The model under review builds one solid part; all positions refer to its coordinate system, in mm. Give positions to 0.01 mm unless a question says otherwise; leave off trailing zeros. Order: outer loops, then holes, each group sorted by start corner. A loop starts at its lowest first (then second) coordinate and runs counter-clockwise, first axis right, second up. Notation, with made-up numbers: (86, 39.25) - (134, 39.25) arc R27 cw to (134, 55.25) - close; hole circle Ø3 at (81, -38.75). An arc over 180 degrees is marked (long way). Use a Markdown table: item, result. Add a question column.
Autodesk Fusion 360 part; units mm, degrees
sketch "草图1" plane through (0, 0, 0) normal (0, 1, 0) x (1, 0, 0)
  line L0 (-18.7279, -36.0337) -> (2.3028, -15.3397)
  line L1 (2.3028, -15.3397) -> (28.4829, -28.9463)
  line L2 (28.4829, -28.9463) -> (15.3006, -2.5501)
  line L3 (15.3006, -2.5501) -> (36.3313, 18.1439)
  line L4 (7.1534, 13.7637) -> (36.3313, 18.1439)
  line L5 (7.1534, 13.7637) -> (-6.0289, 40.1599)
  line L6 (-6.0289, 40.1599) -> (-10.8795, 11.0565)
  line L7 (-40.0574, 6.6762) -> (-10.8795, 11.0565)
  line L8 (-40.0574, 6.6762) -> (-13.8773, -6.9304)
  line L9 (-13.8773, -6.9304) -> (-18.7279, -36.0337)
  line L10 (-30.4812, 5.0802) -> (-12.8573, 7.726)
  line L11 (10.0219, 11.1607) -> (27.6459, 13.8065)
  line L12 (-4.5877, 30.5593) -> (-7.5175, 12.9803)
  line L13 (-11.321, -9.8405) -> (-14.2508, -27.4195)
  line L14 (-30.4812, 5.0802) -> (-14.668, -3.1384)
  line L15 (5.8605, -13.8078) -> (21.6738, -22.0264)
  line L16 (-14.2508, -27.4195) -> (-1.5478, -14.9199)
  line L17 (14.943, 1.3069) -> (27.6459, 13.8065)
  line L18 (21.6738, -22.0264) -> (13.7114, -6.0826)
  line L19 (3.3747, 14.6154) -> (-4.5877, 30.5593)
  circle A0 centre (0, 0) radius 11
  arc A1 (-12.8573, 7.726) -> (-14.668, -3.1384) centre (0, 0) ccw
  arc A2 (3.3747, 14.6154) -> (-7.5175, 12.9803) centre (0, 0) ccw
  arc A3 (14.943, 1.3069) -> (10.0219, 11.1607) centre (0, 0) ccw
  arc A4 (-11.321, -9.8405) -> (-1.5478, -14.9199) centre (0, 0) ccw
  arc A5 (5.8605, -13.8078) -> (13.7114, -6.0826) centre (0, 0) ccw
  dimension "d3" = 30
  dimension "d8" = 22
sketch "草图3" plane through (0, 0, 0) normal (0, 1, 0) x (1, 0, 0)
  circle A0 centre (-75, 0) radius 2.5
  circle A1 centre (-75, 0) radius 4
  dimension "d4" = 5
  dimension "d5" = 8
extrude "拉伸1" add sketch "草图3" along normal blind 3 makes body 1
extrude "拉伸2" add sketch "草图1" along normal blind 3 separate body makes body 2
move_body "移动1" bodies 1 to x (1, 0, 0) y (0, 1, 0) z (0, 0, 1) at (69.0763, 0, -40.5763)
move_body "移动2" bodies 1 to x (1, 0, 0) y (0, 1, 0) z (0, 0, 1) at (-0.4652, 0, -2.1709)
combine "合并1" operation add target body 2 tool bodies 1
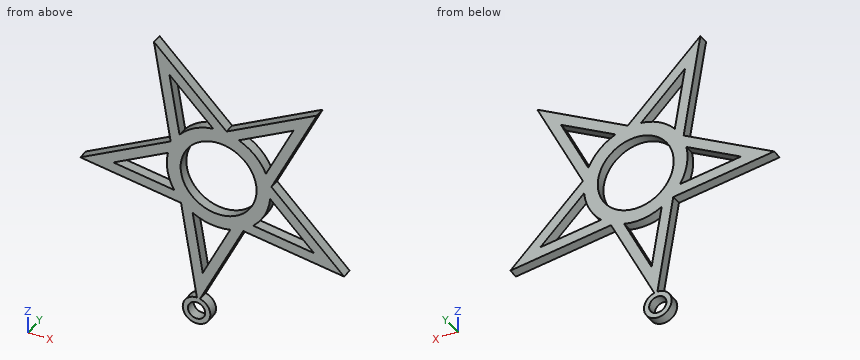
Q1. We need section C-C (z = 0). Write out the cut boundary in (x, y), plus the area to 3 significant figures.
Q2. We need section D-D (z = 16.5). Write out the cut boundary in (x, y).
Q3. We need section B-B (x = 0). Write out the cut boundary in (y, z).
Q4. Clearance check with flat-ended pins moving along their axes: P1, Ø17.5, axis at x = 0, z = 0, coming from the +Y side; P2, Ø1, axis at x = 5, y = 0.5, coming from the +Z side; P3, Ø1, axis at x = 15, y = 0.5, coming from the +Z side. State where each tip first meets the part, or that it passes through.
Q5. Wall thickness on probe 1 along Z at (x, y) = (6.5, 2.65); probe 2 along X at (y, z) = (0.85, 20); probe 3 along Z at (x, y) = (25.5, 1.8): over which ranges is each line inside the solid? List them lowest first.
Q6. We need section A-A (z = -25.5). Write out the cut boundary in (x, y), plus the area to 3 significant figures.
Here are the results:
| question | item | result |
|---|---|---|
| 1 | outline | (-27.21, 0) - (-20.71, 0) - (-20.71, 3) - (-27.21, 3) - close; (-15, 0) - (-11, 0) - (-11, 3) - (-15, 3) - close; (11, 0) - (17.89, 0) - (17.89, 3) - (11, 3) - close |
| 1 | area | 52.2 mm2 |
| 2 | outline | (-15.47, 0) - (-12.43, 0) - (-12.43, 3) - (-15.47, 3) - close; (-3.15, 0) - (1.12, 0) - (1.12, 3) - (-3.15, 3) - close; (4.54, 0) - (11.04, 0) - (11.04, 3) - (4.54, 3) - close; (18.91, 0) - (22.27, 0) - (22.27, 3) - (18.91, 3) - close |
| 3 | outline | (0, -28.09) - (3, -28.09) - (3, -21.37) - (0, -21.37) - close; (0, -15) - (3, -15) - (3, -11) - (0, -11) - close; (0, 11) - (3, 11) - (3, 17.61) - (0, 17.61) - close |
| 4 | P1 | through |
| 4 | P2 | z = 17 |
| 4 | P3 | z = 22.2 |
| 5 | probe 1 | -15.07 to -8.87, 8.87 to 13.52, 14.14 to 17.52 |
| 5 | probe 2 | -16.06 to -13.01, -6.71 to -2.43, 11.27 to 17.77, 20.66 to 24.02 |
| 5 | probe 3 | -16.52 to -13.48, -11.69 to -7.49, 22.97 to 27.4 |
| 6 | outline | (-8.47, 0) - (-5.43, 0) - (-5.43, 3) - (-8.47, 3) - close; (-2.06, 0) - (1.29, 0) - (1.29, 3) - (-2.06, 3) - close |
| 6 | area | 19.2 mm2 |
